```python
from build123d import *

# Parameters (mm, degrees)
SKETCH_1_W          = 250
SKETCH_1_H          = 60
EXTRUDE_1_DEPTH     = 10
SKETCH_8_W          = 10
SKETCH_8_H          = 10
CUT_EXTRUDE_3_DEPTH = 10
CUT_EXTRUDE_4_DEPTH = 10
CUT_EXTRUDE_5_DEPTH = 10


with BuildPart() as part:
    # 草图1 → 凸台-拉伸1 (new body)
    with BuildSketch(Plane.XY):
        with Locations((-17.927308448, 36.060903733)):
            Rectangle(SKETCH_1_W, SKETCH_1_H)
    extrude(amount=EXTRUDE_1_DEPTH)

    # 草图8 → 切除-拉伸3 (cut)
    with BuildSketch(Plane.ZY.offset(142.927308448)):
        with Locations((5, 36.060903733)):
            Rectangle(SKETCH_8_W, SKETCH_8_H)
    extrude(amount=-CUT_EXTRUDE_3_DEPTH, mode=Mode.SUBTRACT)

    # 草图9 → 切除-拉伸4 (cut)
    with BuildSketch(Plane.XY.offset(10)):
        Polygon((-142.927308448, 41.060903733), (-132.927308448, 51.060903733), (-132.927308448, 41.060903733), align=None)
    extrude(amount=-CUT_EXTRUDE_4_DEPTH, mode=Mode.SUBTRACT)

    # 草图10 → 切除-拉伸5 (cut)
    with BuildSketch(Plane.XY.offset(10)):
        Polygon((-142.927308448, 31.060903733), (-132.927308448, 21.060903733), (-132.927308448, 31.060903733), align=None)
    extrude(amount=-CUT_EXTRUDE_5_DEPTH, mode=Mode.SUBTRACT)


solid = part.part
```
The model under review builds one solid part; all positions refer to its coordinate system, in mm. A direction names the side the tool comes from. Round coordinates to 2 decimals unless told otherwise and drop trailing zeros. Loops run counter-clockwise (first coordinate to the right, second up) from the corner with the lowest first, then second, coordinate; pieces in that order, holes last. Notation, with made-up numbers: M 27,24.5 L 78,24.5 A27 ccw 78,49.5 Z; hole C -14,-26.75 d7. An arc over 180 degrees is marked long. Answer as a JSON object with one key per item and string values.
(1) To check wall thickness, follow line 1 along X through (y, z) = (46.5, 8.5); line 2 along X through (y, z) = (48, 7.5); line 3 along X through (y, z) = (31.5, 4.75). State the ranges of each line that lie inside material, in increasing order.
Resolved:
{"line 1": "-142.93 to -137.49, -132.93 to 107.07", "line 2": "-142.93 to -135.99, -132.93 to 107.07", "line 3": "-132.93 to 107.07"}
(2) Take a section at A-A on y = 37. Give the boundary of the cut face in (x, z), and give its area (3 significant figures).
Resolved:
{"outline": "M -132.93,0 L 107.07,0 L 107.07,10 L -132.93,10 Z", "area": "2,400 mm²"}
(3) Tool access review of faces 5 (the flat face through (-132.927, 36, 5)), 6 (the flat face through (-20, 36, 10)): name each direction out of +Z, -Z, +X, -X, +Y, -Y from which nothing blocks a thin tool from reaching the whole face with its end or side.
Resolved:
{"face 5": "+Z, -Z", "face 6": "+Z, +X, -X, +Y, -Y"}
(4) Draft analysis for pull direction Y (two halves, no side actions). For faces 1 (the flat face through (-137.997, 26.131, 5.07)), 2 (the flat face through (-142.927, 53, 5)), 3 (the flat face through (-20, 6.061, 5)), 4 (the flat face through (-20, 66.061, 5)), state which applies: released by +Y, released by -Y, zero draft, split by the parting line, or undercut.
Resolved:
{"face 1": "undercut", "face 2": "zero draft", "face 3": "released by -Y", "face 4": "released by +Y"}
